Model file for the job. Use its own axes, mm. A direction names the side the tool comes from. Coordinates: 2 decimals unless noted, no trailing zeros. Write each loop counter-clockwise with the first axis right and the second up, starting at its lowest first coordinate (ties: lowest second). Pieces come first, ordered by that corner, then holes. Notation, with made-up numbers: M 81.5,40 L 114.5,40 A18 cw 114.5,65 Z; hole C -1,-20.5 d3. An arc over 180 degrees is marked long. Use CSV: the item, a comma, the result in double quotes. Start each with the question number.
from build123d import *

# Parameters (mm, degrees)
BOSS_EXTRUDE1_DEPTH = 13
FILLET1_R           = 1
FILLET2_R           = 10
SKETCH4_R           = 2.355
SKETCH4_W           = 1.42
SKETCH4_H           = 6.26
CUT_EXTRUDE1_DEPTH  = 18


with BuildPart() as part:
    # Sketch1 → Boss-Extrude1 (new body)
    with BuildSketch(Plane(origin=(0, 0, 0), x_dir=(0, 0, -1), z_dir=(1, 0, 0))):
        with BuildLine():
            Line((-8.5, 7.935), (8.5, 7.935))
            Line((8.5, 7.935), (8.5, -1.065))
            Line((8.5, -1.065), (7, -1.065))
            Line((7, -1.065), (3.722478373, -9.398951763))
            ThreePointArc((3.722478373, -9.398951763), (0, -11.935), (-3.722478373, -9.398951763))
            Line((-3.722478373, -9.398951763), (-7, -1.065))
            Line((-7, -1.065), (-8.5, -1.065))
            Line((-8.5, -1.065), (-8.5, 7.935))
        make_face()
    extrude(amount=-BOSS_EXTRUDE1_DEPTH)

    # Fillet1
    fillet1_edges = [part.edges().sort_by_distance(p)[0] for p in [
        (-6.5, 7.935, 8.5),
        (-6.5, 7.935, -8.5),
        (-6.5, -1.065, -8.5),
        (-6.5, -1.065, 8.5),
    ]]
    fillet(fillet1_edges, radius=FILLET1_R)

    # Fillet2
    fillet2_edges = [part.edges().sort_by_distance(p)[0] for p in [
        (-6.5, -1.065, -7),
        (-6.5, -1.065, 7),
    ]]
    fillet(fillet2_edges, radius=FILLET2_R)

    # Sketch4 → Cut-Extrude1 (cut)
    with BuildSketch(Plane.ZY.offset(13)):
        with Locations((0, -8.06)):
            Circle(SKETCH4_R)
        with Locations((6.24, 3.805)):
            Rectangle(SKETCH4_W, SKETCH4_H)
        with Locations((-6.24, 3.805)):
            Rectangle(SKETCH4_W, SKETCH4_H)
    extrude(amount=-CUT_EXTRUDE1_DEPTH, mode=Mode.SUBTRACT)


solid = part.part
1) Band-saw the part on B-B on y = 4. List the corners of the cut face in (x, z).
2) Drop flat-ended pins along their axis: P1, Ø1.6, axis at x = -8.5, z = 6.5, coming from the -Y side; P2, Ø6, axis at x = -6.5, z = 5, coming from the -Y side. Give the stop position or say it passes through.
3) Band-saw the part on C-C on y = -8.06. List the corners of the cut face in (x, z) (3 decimals), then the cut area to 3 significant figures.
4) Band-saw the part on A-A on z = 0. List the corners of the cut face in (x, y) (3 decimals), then the cut area to 3 significant figures.
5) Band-saw the part on D-D on x = -1.75. State how many separate pieces and enclosed holes the cut face has, then the cut area to 3 significant figures.
6) Wall check: L1, parallel to Z at x = -5.25, y = 1.25; L2, parallel to Y at x = -7.5, z = 0 (3 decimals); L3, parallel to Z at x = -1.25, y = -8. Give the ranges that are in metal, low to high. Write a range as [from, to].
7) Two-plate mould, pull along Y, no slides. Class faces 1 (the face through (-7, 4, -6.95)), 2 (the face through (0, 0, 0)), 3 (the face through (-6.409, -6.979, 4.674)), 4 (the face through (-7, 6.935, 6)): pulls with the +Y half, pulls with the -Y half, needs draft (parallel to the pull), parting line crosses it, or undercut.
8) Tool access for faces 5 (the face through (-6.59, 7.65, -8.2)), 6 (the face through (-7, 4, 5.53)): list every direction of +Z, -Z, +X, -X, +Y, -Y with a clear straight run to the whole face (end or side of a thin tool).
Findings below:
1,outline,"M -13,-8.5 L 0,-8.5 L 0,-6.95 L -13,-6.95 Z; M -13,-5.53 L 0,-5.53 L 0,5.53 L -13,5.53 Z; M -13,6.95 L 0,6.95 L 0,8.5 L -13,8.5 Z"
2,P1,"stops at y = -4.37"
2,P2,"stops at y = -11.4"
3,outline,"M -13,-4.249 L 0,-4.249 L 0,-2.355 L -13,-2.355 Z; M -13,2.355 L 0,2.355 L 0,4.249 L -13,4.249 Z"
3,area,"49.2 mm2"
4,outline,"M -13,-11.935 L 0,-11.935 L 0,-10.415 L -13,-10.415 Z; M -13,-5.705 L 0,-5.705 L 0,7.935 L -13,7.935 Z"
4,area,"197 mm2"
5,separate pieces,"1"
5,enclosed holes,"3"
5,area,"222 mm2"
6,L1,"z = [-8.5, -6.95], [-5.53, 5.53], [6.95, 8.5]"
6,L2,"y = [-11.935, -10.415], [-5.705, 7.935]"
6,L3,"z = [-4.27, -2.35], [2.35, 4.27]"
7,face 1,"undercut"
7,face 2,"needs draft"
7,face 3,"pulls with the -Y half"
7,face 4,"undercut"
8,face 5,"-Z, +X, -X, +Y"
8,face 6,"+X, -X"
